Build history of the part. All positions in model axes, mm. Face numbers are marked on the shaded views. A direction names the side the tool comes from. Give positions to 0.01 mm unless a question says otherwise; leave off trailing zeros. Order: outer loops, then holes, each group sorted by start corner. A loop starts at its lowest first (then second) coordinate and runs counter-clockwise, first axis right, second up. Notation, with made-up numbers: (28.25, 75) -> (75.25, 75) arc R34 cw to (75.25, 110) -> close; hole circle Ø6 at (-26, -21). An arc over 180 degrees is marked (long way). One line per question, with ' | ' between items. Start each with the question number.
(1) Drill centre lines: L1, parallel to Y at x = 17.5, z = 29.5; L2, parallel to Y at x = 1, z = 27.5; L3, parallel to X at y = 3.5, z = 11. Where is each one in solid material? Low to high. Write a range as from..to.
(2) Cut at B-B (y = -31.5). Give the cut face in (x, z), then the cut area to 3 significant figures.
(3) Which spindle directions (+Z, -Z, +X, -X, +Y, -Y) get a long thin tool onto all of the face, cutting with end or side? Do the marked faces 4 and 5. Say none if no direction does.
(4) Cut at A-A (z = 23). Give the number of separate pieces and of enclosed holes in the cut face, then the cut area to 3 significant figures.
(5) Pull direction X, two halves, no side cores. Call the marked faces 1, 2 and 3: +X half, -X half, draft (parallel to the pull), parting line (faces both ways), or undercut.
(6) Cut at D-D (x = -6.5). Give the cut face in (y, z), then the cut area to 3 significant figures.
(7) Cut at C-C (x = -16.5). Give the cut face in (y, z).
(8) Pin check, flat tip, straight feed: pin 1 Ø20.5 at (x, y) = (-0.5, -16) entering from +Z. Stop position of the tip, or through.
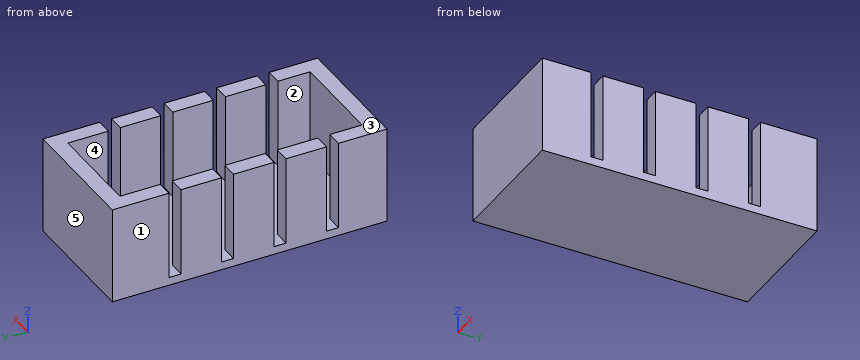
from build123d import *

# Parameters (mm, degrees)
F0_W     = 40.64
F0_H     = 86.36
F0_W_2   = 30.48
F0_H_2   = 76.2
F1_DEPTH = 30.48
F2_DEPTH = 2.54
F3_W     = 5.08
F3_H     = 3.81
F4_DEPTH = 27.94


# Not quite as in the source:
# - a feature names something its author has since deleted; it is built from what else it names


with BuildPart() as f1:
    # F0 (on Top) → F1 (new body)
    with BuildSketch(Plane.XY):
        Rectangle(F0_W, F0_H)
        Rectangle(F0_W_2, F0_H_2, mode=Mode.SUBTRACT)
    extrude(amount=F1_DEPTH)

    # F0 (on Top) → F2 (join)
    with BuildSketch(Plane.XY):
        Rectangle(F0_W_2, F0_H_2)
    extrude(amount=F2_DEPTH)

    # F3 (on face) → F4 (cut)
    with BuildSketch(Plane.XY.offset(30.48)):
        with Locations((-17.78, 23.495)):
            Rectangle(F3_W, F3_H)
        with Locations((17.78, 23.495)):
            Rectangle(F3_W, F3_H)
        with Locations((17.78, 6.985)):
            Rectangle(F3_W, F3_H)
        with Locations((-17.78, 6.985)):
            Rectangle(F3_W, F3_H)
        with Locations((-17.78, -9.525)):
            Rectangle(F3_W, F3_H)
        with Locations((17.78, -9.525)):
            Rectangle(F3_W, F3_H)
        with Locations((-17.78, -26.035)):
            Rectangle(F3_W, F3_H)
        with Locations((17.78, -26.035)):
            Rectangle(F3_W, F3_H)
    extrude(amount=-F4_DEPTH, mode=Mode.SUBTRACT)


solid = f1.part
Result set:
1) L1: y = -43.18..-27.94, -24.13..-11.43, -7.62..5.08, 8.89..21.59, 25.4..43.18 | L2: y = -43.18..-38.1, 38.1..43.18 | L3: x = -20.32..-15.24, 15.24..20.32
2) outline: (-20.32, 0) -> (20.32, 0) -> (20.32, 30.48) -> (15.24, 30.48) -> (15.24, 2.54) -> (-15.24, 2.54) -> (-15.24, 30.48) -> (-20.32, 30.48) -> close | area: 387 mm2
3) face 4: +Z | face 5: +Z, -Z, +X, -X, +Y
4) separate pieces: 8 | enclosed holes: 0 | area: 1,030 mm2
5) face 1: -X half | face 2: undercut | face 3: draft
6) outline: (-43.18, 0) -> (43.18, 0) -> (43.18, 30.48) -> (38.1, 30.48) -> (38.1, 2.54) -> (-38.1, 2.54) -> (-38.1, 30.48) -> (-43.18, 30.48) -> close | area: 503 mm2
7) outline: (-43.18, 0) -> (43.18, 0) -> (43.18, 30.48) -> (25.4, 30.48) -> (25.4, 2.54) -> (21.59, 2.54) -> (21.59, 30.48) -> (8.89, 30.48) -> (8.89, 2.54) -> (5.08, 2.54) -> (5.08, 30.48) -> (-7.62, 30.48) -> (-7.62, 2.54) -> (-11.43, 2.54) -> (-11.43, 30.48) -> (-24.13, 30.48) -> (-24.13, 2.54) -> (-27.94, 2.54) -> (-27.94, 30.48) -> (-43.18, 30.48) -> close
8) pin 1: stops at z = 2.54
